Geometry: final body of the model. Coordinates: model frame, mm. A direction names the side the tool comes from. Give positions to 0.01 mm unless a question says otherwise; leave off trailing zeros. Order: outer loops, then holes, each group sorted by start corner. A loop starts at its lowest first (then second) coordinate and runs counter-clockwise, first axis right, second up. Notation, with made-up numbers: (80, 22.25) -> (130, 22.25) arc R20 cw to (130, 57.25) -> close; hole circle Ø4 at (81, 19.5). An arc over 180 degrees is marked (long way). Answer in a Markdown table with one row per item. Add a question column.
Q1. Line query: line 1 along Y through (x, z) = (16, -10.5); line 2 along Z through (x, y) = (75, -1.5); line 3 along Y through (x, z) = (-2.5, -15.5). Output: solid intervals per line, ascending. Write a range as from..to.
Q2. Cut plane A-A on x = 45.5. Return the cut outline in (y, z), and give its area (3 significant figures).
Q3. Cut plane B-B on z = 8.5. Return the cut outline in (x, y), and give its area (3 significant figures).
Q4. Cut plane C-C on y = -50. Return the cut outline in (x, z).
Q5. Cut plane D-D on z = -4. Return the cut outline in (x, y), and give its area (3 significant figures).
Q6. Pull-direction query (Z, two-part tool) for faces 5 (the face through (22, 10, 0)), 6 (the face through (69, 6, 18)), 7 (the face through (81.51, 1.69, -16.47)), 8 (the face through (74, 5, 19)); classes: +Z half, -Z half, draft (parallel to the pull), parting line (faces both ways), or undercut.
Q7. Contact query for flat-ended pins moving along their axis: P1, Ø0.8, axis at x = 64.5, z = -18.5, coming from the -Y side; P2, Ø11.5, axis at x = 56, z = 7.5, coming from the -Y side; P3, Ø21.5, axis at x = 40.5, y = -34.5, coming from the -Z side; P4, Ø1, axis at x = 80.5, y = 3.5, coming from the -Z side. Output: stop coordinate, or through.
Q8. Set-up query: faces 1 (the face through (24, 10, -17)), 2 (the face through (63, 10, 11.995)), 3 (the face through (73, 2.1, 18.5)), 4 (the face through (29.7, -22.2, -16)). Return all of +Z, -Z, +X, -X, +Y, -Y with unobstructed straight access to the full face (end or side cutting, diameter ignored); none if empty.
from build123d import *

# Parameters (mm, degrees)
F1_DEPTH  = 16
F2_W      = 70
F2_H      = 3
F3_DEPTH  = 2
F4_W      = 50
F4_H      = 14
F5_DEPTH  = 1
F6_R      = 1
F9_DEPTH  = 2
F11_DEPTH = 1.001
F13_D     = 4
F13_DEPTH = 50
F13_TIP   = 1.2017212381
F14_R     = 3
F14_R_2   = 2
F15_DEPTH = 5
F16_R     = 3
F18_D     = 4
F18_DEPTH = 50
F18_TIP   = 1.2017212381


# Not quite as in the source:
# - a pattern or mirror of a feature is missing from the dataset's text; its kind, count and spacing are read off the source's solid


with BuildPart() as f1:
    # F0 (on Top) → F1 (new body)
    with BuildSketch(Plane.XY):
        with BuildLine():
            Line((94, 11), (0, 11))
            ThreePointArc((0, 11), (-11, 0), (0, -11))
            Line((0, -11), (19, -11))
            ThreePointArc((19, -11), (21.7681124643, -11.8361612201), (23.6103896104, -14.064978646))
            ThreePointArc((23.6103896104, -14.064978646), (46.8644288503, -43.8489365308), (81.9993431207, -57.7547729841))
            ThreePointArc((81.9993431207, -57.7547729841), (87.0632727772, -58.5972193444), (91.5997631119, -61))
            Line((91.5997631119, -61), (94.3248553538, -61))
            ThreePointArc((94.3248553538, -61), (89.9506080698, -57.6601123846), (84.7034264019, -56))
            ThreePointArc((84.7034264019, -56), (49.0672193413, -42.9854179344), (25.4545454545, -13.2909701044))
            ThreePointArc((25.4545454545, -13.2909701044), (22.87535745, -10.1706257081), (19, -9))
            Line((19, -9), (0, -9))
            ThreePointArc((0, -9), (-9, 0), (0, 9))
            Line((0, 9), (94, 9))
            Line((94, 9), (94, 11))
        make_face()
    extrude(amount=F1_DEPTH)

    # F2 (on face) → F3 (join)
    with BuildSketch(Plane(origin=(0, 11, 0), x_dir=(-1, 0, 0), z_dir=(0, 1, 0))):
        with Locations((-59, 17.5)):
            Rectangle(F2_W, F2_H)
    extrude(amount=-F3_DEPTH)

    # F4 (on face) → F5 (join)
    with BuildSketch(Plane.XY.offset(19)):
        with Locations((69, 4)):
            Rectangle(F4_W, F4_H)
    extrude(amount=-F5_DEPTH)

    # F6
    f6_edges = [f1.edges().sort_by_distance(p)[0] for p in [
        (59, 11, 19),
    ]]
    fillet(f6_edges, radius=F6_R)

    # F7: F1 across face


with BuildPart() as f1_1:
    add(f1.part)
    add(f1.part.mirror(Plane(origin=(39.0198924269, -12.8147332924, 0), x_dir=(1, 0, 0), z_dir=(0, 0, -1))))

    # F8 (on face) → F9 (cut)
    with BuildSketch(Plane(origin=(0, 11, 0), x_dir=(-1, 0, 0), z_dir=(0, 1, 0))):
        with BuildLine():
            Line((-94, -12), (-34, -12))
            ThreePointArc((-34, -12), (-22.001130085, -0.1646838272), (-33.6706633635, 11.9954798728))
            Line((-33.6706633635, 11.9954798728), (-34.3293366365, 11.9954798728))
            Line((-34.3293366365, 11.9954798728), (-94, 11.9954798728))
            Line((-94, 11.9954798728), (-94, -12))
        make_face()
    extrude(amount=-F9_DEPTH, mode=Mode.SUBTRACT)

    # F10 (on face) → F11 (cut, through all)
    with BuildSketch(Plane(origin=(0, 0, 18), x_dir=(1, 0, 0), z_dir=(0, 0, -1))):
        with BuildLine():
            ThreePointArc((50, 1), (47, -2), (50, -5))
            Line((50, -5), (70, -5))
            ThreePointArc((70, -5), (73, -2), (70, 1))
            Line((70, 1), (50, 1))
        make_face()
    f11 = extrude(amount=-F11_DEPTH, mode=Mode.SUBTRACT)

    # F11_copies: F11 across plane
    add(f11.mirror(Plane(origin=(0, 0, 0), x_dir=(-1, 0, 0), z_dir=(0, 0, -1))), mode=Mode.SUBTRACT)

    # F13 (one way)
    with BuildSketch(Plane.XY.offset(18)):
        with Locations((80, 3)):
            Circle(F13_D / 2)
    extrude(amount=-F13_DEPTH, mode=Mode.SUBTRACT)
    with Locations(Plane.XY.offset(18)):
        with Locations((80, 3)):
            with Locations((0, 0, -(F13_DEPTH + F13_TIP / 2))):  # 118° drill point
                Cone(0, F13_D / 2, F13_TIP, mode=Mode.SUBTRACT)

    # F14 (on face) → F15 (join)
    with BuildSketch(Plane.XY.offset(19)):
        with Locations((80, 3)):
            Circle(F14_R)
        with Locations((80, 3)):
            Circle(F14_R_2, mode=Mode.SUBTRACT)
    f15 = extrude(amount=-F15_DEPTH)

    # F15_copies: F15 across plane
    add(f15.mirror(Plane(origin=(0, 0, 0), x_dir=(-1, 0, 0), z_dir=(0, 0, -1))))

    # F16
    f16_edges = [f1_1.edges().sort_by_distance(p)[0] for p in [
        (94, -3, 18.5),
        (44, -3, 18.5),
        (44, -3, -18.5),
        (94, -3, -18.5),
    ]]
    fillet(f16_edges, radius=F16_R)

    # F18
    with Locations(Plane.XY.offset(19)):
        with Locations((79.9801871181, 3.0164394993)):
            Hole(F18_D / 2, depth=F18_DEPTH)
            with Locations((0, 0, -(F18_DEPTH + F18_TIP / 2))):  # 118° drill point
                Cone(0, F18_D / 2, F18_TIP, mode=Mode.SUBTRACT)


solid = f1_1.part
Completed:
| question | item | result |
|---|---|---|
| 1 | line 1 | y = -11..-9, 9..11 |
| 1 | line 2 | z = -19..-18, 18..19 |
| 1 | line 3 | y = -10.71..-8.65, 8.65..10.71 |
| 2 | outline | (-42.8, -16) -> (-40.24, -16) -> (-40.24, 16) -> (-42.8, 16) -> close; (-2.6, -19) -> (10, -19) arc R1 ccw to (11, -18) -> (11, -12) -> (9, -12) -> (9, -18) -> (-2.6, -18) -> close; (-2.6, 18) -> (9, 18) -> (9, 12) -> (11, 12) -> (11, 18) arc R1 ccw to (10, 19) -> (-2.6, 19) -> close |
| 2 | area | 133 mm² |
| 3 | outline | (0, -11) -> (19, -11) arc R5 cw to (23.61, -14.06) arc R72 ccw to (82, -57.75) arc R16 cw to (91.6, -61) -> (94.32, -61) arc R16 ccw to (84.7, -56) arc R70 cw to (25.45, -13.29) arc R7 ccw to (19, -9) -> (0, -9) arc R9 cw to (0, 9) -> (25.53, 9) -> (25.53, 11) -> (0, 11) arc R11 ccw to start |
| 3 | area | 340 mm² |
| 4 | outline | (56.63, -16) -> (61.2, -16) -> (61.2, 16) -> (56.63, 16) -> close |
| 5 | outline | (0, -11) -> (19, -11) arc R5 cw to (23.61, -14.06) arc R72 ccw to (82, -57.75) arc R16 cw to (91.6, -61) -> (94.32, -61) arc R16 ccw to (84.7, -56) arc R70 cw to (25.45, -13.29) arc R7 ccw to (19, -9) -> (0, -9) arc R9 cw to (0, 9) -> (22.69, 9) -> (22.69, 11) -> (0, 11) arc R11 ccw to start |
| 5 | area | 334 mm² |
| 6 | face 5 | undercut |
| 6 | face 6 | undercut |
| 6 | face 7 | draft |
| 6 | face 8 | +Z half |
| 7 | P1 | stops at y = -3 |
| 7 | P2 | stops at y = -52.43 |
| 7 | P3 | stops at z = -16 |
| 7 | P4 | passes through |
| 8 | face 1 | -Z, -X, +Y, -Y |
| 8 | face 2 | +X, +Y |
| 8 | face 3 | +Z, -Z |
| 8 | face 4 | -Z, -X, -Y |
